Geometry: final body of the model. Coordinates: model frame, mm. Coordinates: 2 decimals unless noted, no trailing zeros. Write each loop counter-clockwise with the first axis right and the second up, starting at its lowest first coordinate (ties: lowest second). Pieces come first, ordered by that corner, then holes. Notation, with made-up numbers: (11.5, 34.25) -> (57.5, 34.25) arc R12 cw to (57.5, 40.25) -> close; hole circle Ø7 at (-6, 60). An arc over 180 degrees is marked (long way). Answer as a JSON object with one key per item and string values. Group by question number.
```python
from build123d import *

# Parameters (mm, degrees)
SKETCH1_W           = 50.292
SKETCH1_H           = 43
SKETCH1_R           = 7.5
BOSS_EXTRUDE1_DEPTH = 1.6
SKETCH2_R           = 1.3
CUT_EXTRUDE3_DEPTH  = 2.6


with BuildPart() as part:
    # Sketch1 → Boss-Extrude1 (new body)
    with BuildSketch(Plane(origin=(0, 0, 0), x_dir=(1, 0, 0), z_dir=(0, 1, 0))):
        Rectangle(SKETCH1_W, SKETCH1_H)
        Circle(SKETCH1_R, mode=Mode.SUBTRACT)
    extrude(amount=BOSS_EXTRUDE1_DEPTH)

    # Sketch2 → Cut-Extrude3 (cut, through all)
    with BuildSketch(Plane(origin=(0, 0, 0), x_dir=(1, 0, 0), z_dir=(0, 1, 0))):
        with Locations((-14, 17.5)):
            Circle(SKETCH2_R)
        with Locations((14, 17.5)):
            Circle(SKETCH2_R)
        with Locations((14, -17.5)):
            Circle(SKETCH2_R)
        with Locations((-14, -17.5)):
            Circle(SKETCH2_R)
    extrude(amount=CUT_EXTRUDE3_DEPTH, mode=Mode.SUBTRACT)


solid = part.part
```
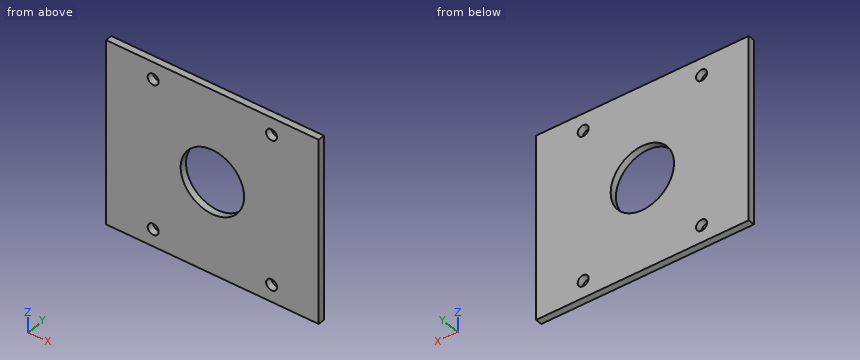
Item 1: Section B-B on x = 0. Output: boundary loops of the cut face in (y, z), then the cut area to 3 significant figures.
Item 2: Section A-A on z = -17.5. Output: boundary loops of the cut face in (x, y), then the cut area to 3 significant figures.
Item 3: Section D-D on z = 0. Output: boundary loops of the cut face in (x, y).
Item 4: Ray query, L1, parallel to X at y = 0.5, z = -17.5; L2, parallel to Z at x = 14, y = 0.75; L3, parallel to X at y = 0.7, z = -17. Return the intervals inside material, ascending. Write a range as [from, to].
Item 5: Section C-C on x = -14. Output: boundary loops of the cut face in (y, z), then the cut area to 3 significant figures.
Item 6: Contact query for a flat-ended pin moving along its axis: pin 1 (3 mm diameter, centred on x = -10.5, z = 0.5, fed in from -Y). Output: stop coordinate, or through.
Answer sheet:
{
 "1": {"outline": "(0, -21.5) -> (1.6, -21.5) -> (1.6, -7.5) -> (0, -7.5) -> close; (0, 7.5) -> (1.6, 7.5) -> (1.6, 21.5) -> (0, 21.5) -> close", "area": "44.8 mm^2"},
 "2": {"outline": "(-25.15, 0) -> (-15.3, 0) -> (-15.3, 1.6) -> (-25.15, 1.6) -> close; (-12.7, 0) -> (12.7, 0) -> (12.7, 1.6) -> (-12.7, 1.6) -> close; (15.3, 0) -> (25.15, 0) -> (25.15, 1.6) -> (15.3, 1.6) -> close", "area": "72.1 mm^2"},
 "3": {"outline": "(-25.15, 0) -> (-7.5, 0) -> (-7.5, 1.6) -> (-25.15, 1.6) -> close; (7.5, 0) -> (25.15, 0) -> (25.15, 1.6) -> (7.5, 1.6) -> close"},
 "4": {"L1": "x = [-25.15, -15.3], [-12.7, 12.7], [15.3, 25.15]", "L2": "z = [-21.5, -18.8], [-16.2, 16.2], [18.8, 21.5]", "L3": "x = [-25.15, -15.2], [-12.8, 12.8], [15.2, 25.15]"},
 "5": {"outline": "(0, -21.5) -> (1.6, -21.5) -> (1.6, -18.8) -> (0, -18.8) -> close; (0, -16.2) -> (1.6, -16.2) -> (1.6, 16.2) -> (0, 16.2) -> close; (0, 18.8) -> (1.6, 18.8) -> (1.6, 21.5) -> (0, 21.5) -> close", "area": "60.5 mm^2"},
 "6": {"pin 1": "stops at y = 0"}
}
